from build123d import *

# Parameters (mm, degrees)
SKETCH1_W           = 97
SKETCH1_H           = 97
SKETCH1_W_2         = 72
SKETCH1_H_2         = 72
BOSS_EXTRUDE1_DEPTH = 1
SKETCH2_W           = 10
SKETCH2_H           = 10
CUT_EXTRUDE1_DEPTH  = 69.596647148
FILLET1_R           = 10


with BuildPart() as part:
    # Sketch1 → Boss-Extrude1 (new body)
    with BuildSketch(Plane.XY):
        Rectangle(SKETCH1_W, SKETCH1_H)
        Rectangle(SKETCH1_W_2, SKETCH1_H_2, mode=Mode.SUBTRACT)
    extrude(amount=BOSS_EXTRUDE1_DEPTH)

    # Sketch2 → Cut-Extrude1 (cut, through all)
    with BuildSketch(Plane.XY.offset(1)):
        with Locations((-43.5, 43.5)):
            Rectangle(SKETCH2_W, SKETCH2_H)
        with Locations((43.5, 43.5)):
            Rectangle(SKETCH2_W, SKETCH2_H)
        with Locations((43.5, -43.5)):
            Rectangle(SKETCH2_W, SKETCH2_H)
        with Locations((-43.5, -43.5)):
            Rectangle(SKETCH2_W, SKETCH2_H)
    extrude(amount=-CUT_EXTRUDE1_DEPTH, mode=Mode.SUBTRACT)

    # Fillet1
    fillet1_edges = [part.edges().sort_by_distance(p)[0] for p in [
        (-36, -36, 0.5),
        (-38.5, -38.5, 0.5),
        (38.5, -38.5, 0.5),
        (36, -36, 0.5),
        (38.5, 38.5, 0.5),
        (36, 36, 0.5),
        (-38.5, 38.5, 0.5),
        (-36, 36, 0.5),
    ]]
    fillet(fillet1_edges, radius=FILLET1_R - 0.0001)  # a hair under: the kernel refuses the full size


solid = part.part
Check sheet for the modelled part. Datum: model origin and axes. Units: mm. A direction names the side the tool comes from. Round coordinates to 2 decimals unless told otherwise and drop trailing zeros. Order: outer loops, then holes, each group sorted by start corner. A loop starts at its lowest first (then second) coordinate and runs counter-clockwise, first axis right, second up.
Q1. Cross-section at A-A, the plane x = 3. Enter the section's corners in (y, z).
Filled sheet:
outline: (-48.5, 0) - (-36, 0) - (-36, 1) - (-48.5, 1) - close; (36, 0) - (48.5, 0) - (48.5, 1) - (36, 1) - close
Q2. Scan lines: L1, parallel to X at y = -24, z = 0.1; L2, parallel to X at y = -27.5, z = 0.4. Record each from-to range of solid material in increasing order.
Filled sheet:
L1: x = -48.5 to -36, 36 to 48.5
L2: x = -48.5 to -35.89, 35.89 to 48.5
Q3. Set-up check for faces 1 (the face through (-41.51, 41.35, 0.49)), 2 (the face through (32.99, -33.15, 0.51)): record each of +Z, -Z, +X, -X, +Y, -Y from which the full face is reachable in a straight line by a thin tool's end or side.
Filled sheet:
face 1: +Z, -Z, -X, +Y
face 2: +Z, -Z
Q4. Cross-section at D-D, the plane y = 42.5. Enter the section's corners in (x, z).
Filled sheet:
outline: (-40.5, 0) - (40.5, 0) - (40.5, 1) - (-40.5, 1) - close
Q5. Draft check along X on faces 3 (the face through (41.35, 41.51, 0.49)), 4 (the face through (-36.2, -7, 1)), 5 (the face through (-33.15, 32.99, 0.51)). Enter one of: pulls with the +X half, pulls with the -X half, needs draft (parallel to the pull), parting line crosses it, or undercut.
Filled sheet:
face 3: pulls with the +X half
face 4: needs draft
face 5: undercut
